Input: dimensioned drawing with shaded views. Units: mm. Origin: part minimum x, y, z. A direction names the side the tool comes from. Coordinates: 2 decimals unless noted, no trailing zeros. Write each loop counter-clockwise with the first axis right and the second up, starting at its lowest first coordinate (ties: lowest second). Pieces come first, ordered by that corner, then holes. Notation, with made-up numbers: M -36,-11.5 L -27,-11.5 A16 cw -27,16.5 Z; hole C 21.5,49.25 d5. An arc over 180 degrees is marked long. Write each question's results on one line, items separated by ' | '. Start each with the question number.
1. Section query B-B, the plane z = 47. Output: boundary loops of the cut face in (x, y).
2. First-contact query: pin 1 (20 mm diameter, centred on x = 355.5, y = 7, fed in from -Z); pin 2 (12.5 mm diameter, centred on y = 9, z = 54, fed in from +X); pin 3 (7.5 mm diameter, centred on y = 12, z = 54.5, fed in from -X). Flat tips, straight axial feed; report the tip coordinate or a pass-through.
3. Pull-direction query (Y, two-part tool) for the marked faces 3, 4 and 5; classes: +Y half, -Y half, draft (parallel to the pull), parting line (faces both ways), or undercut.
4. Ray query, probe 1 along Y at (x, z) = (314, 50.5); probe 2 along Y at (x, z) = (358.5, 84); probe 3 along X at (y, z) = (132, 17). Return the intervals inside material, ascending.
5. Section query D-D, the plane y = 132. Output: boundary loops of the cut face in (x, z), and give its area (3 significant figures).
6. Section query C-C, the plane x = 403. Output: boundary loops of the cut face in (y, z), and give its area (4 significant figures).
7. Section query A-A, the plane y = 16. Output: boundary loops of the cut face in (x, z), and give its area (3 significant figures).
8. Set-up query: the marked faces 1 and 2. Return all of +Z, -Z, +X, -X, +Y, -Y with unobstructed straight access to the full face (end or side cutting, diameter ignored); none if empty.
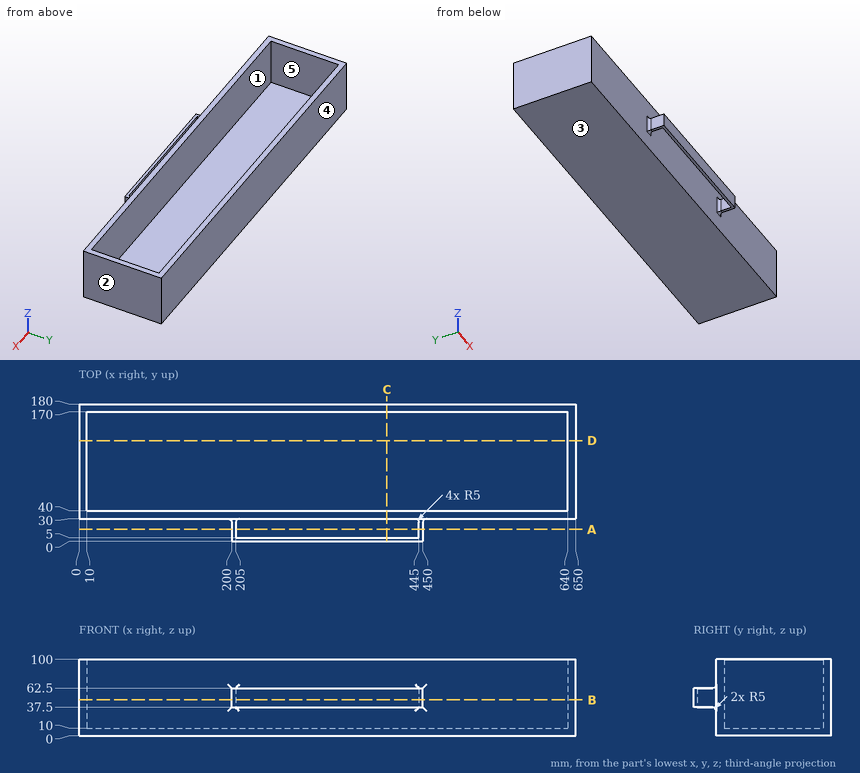
Answer:
1) outline: M 0,30 L 195,30 A5 cw 200,25 L 200,0 L 450,0 L 450,25 A5 cw 455,30 L 650,30 L 650,180 L 0,180 Z; hole M 10,40 L 640,40 L 640,170 L 10,170 Z; hole M 205,5 L 445,5 L 445,25 A5 ccw 440,30 L 210,30 A5 ccw 205,25 Z
2) pin 1: z = 37.5 | pin 2: x = 450 | pin 3: x = 200
3) face 3: draft | face 4: +Y half | face 5: undercut
4) probe 1: 0 to 5, 30 to 40, 170 to 180 | probe 2: 30 to 40, 170 to 180 | probe 3: 0 to 10, 640 to 650
5) outline: M 0,0 L 650,0 L 650,100 L 640,100 L 640,10 L 10,10 L 10,100 L 0,100 Z | area: 8,300 mm^2
6) outline: M 0,37.5 L 5,37.5 L 5,62.5 L 0,62.5 Z; M 30,0 L 180,0 L 180,100 L 170,100 L 170,10 L 40,10 L 40,100 L 30,100 Z | area: 3,425 mm^2
7) outline: M 200,37.5 L 205,37.5 L 205,62.5 L 200,62.5 Z; M 445,37.5 L 450,37.5 L 450,62.5 L 445,62.5 Z | area: 250 mm^2
8) face 1: +Z | face 2: +Z, -Z, +X, +Y, -Y
